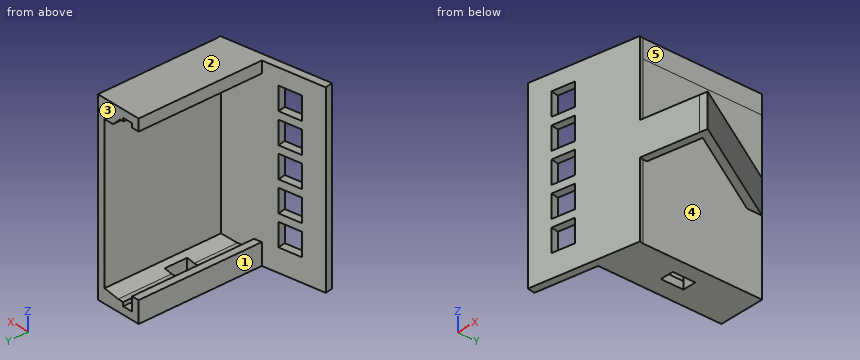
```python
from build123d import *

# Parameters (mm, degrees)
SKETCH1_W           = 38.699948
SKETCH1_H           = 153.19375
BOSS_EXTRUDE1_DEPTH = 0.0254
BOSS_EXTRUDE2_DEPTH = 104.14
SKETCH6_W           = 6.35
SKETCH6_H           = 104.14
BOSS_EXTRUDE3_DEPTH = 119.798010362
BOSS_EXTRUDE7_REACH = 191.252
BOSS_EXTRUDE5_START = -62.626875
BOSS_EXTRUDE5_DEPTH = 27.94
CUT_EXTRUDE1_REACH  = 209.329
SKETCH14_W          = 11.4125
SKETCH14_H          = 19.05
BOSS_EXTRUDE8_REACH = 204.162
SKETCH18_W          = 27.94
SKETCH18_H          = 6.35
SKETCH19_W          = 19.05
SKETCH19_H          = 19.05
CUT_EXTRUDE2_DEPTH  = 208.293560784
SKETCH20_W          = 135.918968774
SKETCH20_H          = 500.058977118
CUT_EXTRUDE3_DEPTH  = 153.162


with BuildPart() as part:
    # Sketch1 → Boss-Extrude1 (new body)
    with BuildSketch(Plane(origin=(0, 0, 0), x_dir=(1, 0, 0), z_dir=(0, 1, 0))):
        with Locations((19.349974, 76.596875)):
            Rectangle(SKETCH1_W, SKETCH1_H)
    extrude(amount=BOSS_EXTRUDE1_DEPTH)

    # Sketch3 → Boss-Extrude2 (add)
    with BuildSketch(Plane(origin=(0, 0.0254, 0), x_dir=(1, 0, 0), z_dir=(0, 1, 0))):
        Polygon((6.15, 146.84375), (14.587499908, 146.84375), (14.587499908, 143.66875), (19.349999908, 143.66875), (32.349999908, 141.684375), (32.349999908, 135.41375), (38.699999908, 135.41375), (38.699999908, 153.19375), (0, 153.19375), (0, 135.41375), (6.15, 135.41375), align=None)
        Polygon((17.762499908, 9.025), (14.587499908, 9.025), (14.587499908, 6.35), (6.15, 6.35), (6.15, 9.74074125), (0, 9.74074125), (0, 0), (38.699921546, 0), (38.699921546, 15.615739638), (24.353239546, 15.615739638), align=None)
    extrude(amount=BOSS_EXTRUDE2_DEPTH)

    # Sketch6 → Boss-Extrude3 (add)
    with BuildSketch(Plane.XY.offset(-135.41375)):
        with Locations((35.524999908, 52.0954)):
            Rectangle(SKETCH6_W, SKETCH6_H)
    extrude(amount=BOSS_EXTRUDE3_DEPTH)

    # Boss-Extrude7: up to this face of the body (flat: up to its plane)
    boss_extrude7_end = Plane(part.part.faces().sort_by_distance((19.349999948, 52.082700017, -153.19375))[0])
    # Sketch15 → Boss-Extrude7 (add, up to the picked face)
    with BuildSketch(Plane.XY, mode=Mode.PRIVATE) as boss_extrude7_sk1:
        Polygon((-50.8, -8.87193717), (-49.680323673, -15.22193717), (39.219676327, 0.453531415), (38.1, 6.803531415), align=None)
    boss_extrude7_tool1 = split(extrude(boss_extrude7_sk1.sketch, amount=-BOSS_EXTRUDE7_REACH, mode=Mode.PRIVATE), bisect_by=boss_extrude7_end, keep=Keep.BOTH, mode=Mode.PRIVATE)
    add(boss_extrude7_tool1.solids().sort_by(Axis((-5.790162, -4.209203, 0), (0, 0, -1)))[0])

    # Sketch11 → Boss-Extrude5 (add)
    with BuildSketch(Plane(origin=(0, 0, -153.19375), x_dir=(-1, 0, 0), z_dir=(0, 0, -1)).offset(BOSS_EXTRUDE5_START)):
        Polygon((-38.699948, 104.1654), (-93.093533667, 9.952946019), (-86.438666859, 8.779513448), (-38.699948, 91.4654), align=None)
    extrude(amount=-BOSS_EXTRUDE5_DEPTH)

    # Sketch14 → Cut-Extrude1 (cut, up to next)
    with BuildSketch(Plane(origin=(0, 0, -153.19375), x_dir=(-1, 0, 0), z_dir=(0, 0, -1)), mode=Mode.PRIVATE) as cut_extrude1_sk1:
        with Locations((-20.293749908, 49.53)):
            Rectangle(SKETCH14_W, SKETCH14_H)
    cut_extrude1_tool1 = extrude(cut_extrude1_sk1.sketch, amount=-CUT_EXTRUDE1_REACH, mode=Mode.PRIVATE) & part.part
    add(cut_extrude1_tool1.solids().sort_by_distance((20.29375, 49.53, -153.19375))[0], mode=Mode.SUBTRACT)

    # Boss-Extrude8: up to this plane
    boss_extrude8_end = Plane(origin=(38.699948, 91.4654, -62.626875), z_dir=(0.8660254037844379, 0.5000000000000011, 0))
    # Sketch18 → Boss-Extrude8 (add, up to the surface)
    with BuildSketch(Plane(origin=(38.114616821, 6.720635305, 0), x_dir=(0, 0, -1), z_dir=(0.9848077530122079, 0.17364817766693177, 0)), mode=Mode.PRIVATE) as boss_extrude8_sk1:
        with Locations((76.596875, -3.188784069)):
            Rectangle(SKETCH18_W, SKETCH18_H)
    boss_extrude8_tool1 = split(extrude(boss_extrude8_sk1.sketch, amount=BOSS_EXTRUDE8_REACH, mode=Mode.PRIVATE), bisect_by=boss_extrude8_end, keep=Keep.BOTH, mode=Mode.PRIVATE)
    add(boss_extrude8_tool1.solids().sort_by_distance((38.668343, 3.580296, -76.596875))[0])

    # Sketch19 → Cut-Extrude2 (cut, through all)
    with BuildSketch(Plane(origin=(-0.014616821, 0.08289611, 0), x_dir=(0.984807753012208, 0.1736481776669311, 0), z_dir=(-0.1736481776669311, 0.984807753012208, 0))):
        with Locations((-22.993829575, 124.61875)):
            Rectangle(SKETCH19_W, SKETCH19_H)
        with Locations((-22.993829575, 99.21875)):
            Rectangle(SKETCH19_W, SKETCH19_H)
        with Locations((-22.993829575, 73.81875)):
            Rectangle(SKETCH19_W, SKETCH19_H)
        with Locations((-22.993829575, 48.41875)):
            Rectangle(SKETCH19_W, SKETCH19_H)
        with Locations((-22.993829575, 23.01875)):
            Rectangle(SKETCH19_W, SKETCH19_H)
    extrude(amount=-CUT_EXTRUDE2_DEPTH, mode=Mode.SUBTRACT)

    # Sketch20 → Cut-Extrude3 (cut)
    with BuildSketch(Plane(origin=(1.105059507, -6.26710389, 0), x_dir=(0.9848077530122079, 0.17364817766693127, 0), z_dir=(0.17364817766693127, -0.9848077530122079, 0))):
        with Locations((20.082569743, -64.610703306)):
            Rectangle(SKETCH20_W, SKETCH20_H)
    extrude(amount=CUT_EXTRUDE3_DEPTH, mode=Mode.SUBTRACT)


solid = part.part
```
Here's how the part is built. I have some questions about the finished solid (model axes, mm). Face numbers are marked on the shaded views. A direction names the side the tool comes from. Give positions to 0.01 mm unless a question says otherwise; leave off trailing zeros. Write each loop counter-clockwise with the first axis right and the second up, starting at its lowest first coordinate (ties: lowest second). Pieces come first, ordered by that corner, then holes. Notation, with made-up numbers: (7, -4.5) -> (30, -4.5) arc R33 ccw to (30, 24.5) -> close; hole circle Ø7 at (-4, 67). An arc over 180 degrees is marked (long way). Write each question's results on one line, items separated by ' | '.
Item 1: Suppose I cut it at B-B on z = -50. Write out the boundary of the cut face in (x, y), plus the area to 3 significant figures.
Output:
outline: (-50.8, -8.87) -> (-49.68, -15.22) -> (-30.92, -11.91) -> (-32.04, -5.56) -> close; (-13.28, -2.26) -> (-12.16, -8.61) -> (39.22, 0.45) -> (38.7, 3.4) -> (38.7, 104.17) -> (32.35, 104.17) -> (32.35, 5.79) -> close | area: 1,080 mm^2
Item 2: If I drill on L1, parallel to Z at x = 14, y = 70; L2, parallel to X at y = 29, z = -42.5; L3, parallel to X at y = 22, z = -83.5, over which ranges is the centre line in solid material (lowest first)?
Output:
L1: z = -153.19 to -146.84, -6.35 to 0 | L2: x = 32.35 to 38.7 | L3: x = 32.35 to 38.7, 78.81 to 86.14
Item 3: We'd pull the mould along X, two halves only. Please class the marked faces 3, 4 and 5: pulls with the +X half, pulls with the -X half, needs draft (parallel to the pull), parting line crosses it, or undercut.
Output:
face 3: needs draft | face 4: undercut | face 5: pulls with the +X half
Item 4: For pin 1 Ø1 at (x, z) = (-2, -73) entering from +Y; pin 2 Ø8 at (y, z) = (62, -123.5) entering from -X; pin 3 Ø2 at (x, y) = (34.5, -3) entering from +Z; pin 4 Ø2.5 at (x, y) = (11, 74) entering from +Z, each with a flat end and sliding along its axis, tell me the tip position at first contact or that it passes through.
Output:
pin 1: stops at y = -0.18 | pin 2: stops at x = 32.35 | pin 3: passes through | pin 4: stops at z = 0
Item 5: Suppose I cut it at A-A on z = -77.5. Give the number of separate pieces and of enclosed holes in the cut face, plus the area to 3 significant figures.
Output:
separate pieces: 2 | enclosed holes: 1 | area: 2,030 mm^2
Item 6: Suppose I cut it at D-D on x = 79. Write out the boundary of the cut face in (y, z), plus the area to 3 significant figures.
Output:
outline: (7.47, -90.57) -> (13.92, -90.57) -> (13.92, -62.63) -> (7.47, -62.63) -> close; (21.66, -90.57) -> (34.36, -90.57) -> (34.36, -62.63) -> (21.66, -62.63) -> close | area: 535 mm^2
Item 7: On a 3-axis mill with a long thin cutter (end or side, diameter ignored), from which of +Z, -Z, +X, -X, +Y, -Y can I reach the whole of each face in a straight line? I mean the marked faces 1 and 2. Say none if no direction works.
Output:
face 1: +Z, -Z, -X, +Y | face 2: +Z, +X, -X, +Y, -Y
